Design review of the part built by this model. Coordinates are the model's own, in mm. A direction names the side the tool comes from. Give positions to 0.01 mm unless a question says otherwise; leave off trailing zeros. Order: outer loops, then holes, each group sorted by start corner. A loop starts at its lowest first (then second) coordinate and runs counter-clockwise, first axis right, second up. Notation, with made-up numbers: (83, 28) -> (121, 28) arc R17 ccw to (121, 49) -> close; hole circle Ø8 at (26, 17). An arc over 180 degrees is marked (long way). One line per item, written item: value. Start each with the question number.
1) Tool access review of faces 3 (the face through (-72.563, -93.809, 13.957)), 4 (the face through (-19.567, 101.123, 20.944)): name each direction out of +Z, -Z, +X, -X, +Y, -Y from which nothing blocks a thin tool from reaching the whole face with its end or side.
2) Consider section A-A (x = 0). State the section outline as (y, z) points, plus the area to 3 significant figures.
3) Consider section B-B (y = 55). State the section outline as (x, z) points.
4) Wall thickness on line 1 along Y through (x, z) = (0, 12.25); line 2 along X through (y, z) = (-3, 4); line 3 along Y through (x, z) = (-20, 10.5): over which ranges is each line inside the solid? List them lowest first. Write a range as from..to.
5) The part is to be moulded in two halves that separate along Y. For faces 1 (the face through (77, -57, 25)), 2 (the face through (-68.887, -95.472, 13.957)), say which applies: released by +Y, released by -Y, zero draft, split by the parting line, or undercut.
6) Consider section C-C (z = 20.5). State how many separate pieces and enclosed holes the cut face has, plus the area to 3 significant figures.
7) For pin 1 (1 mm diameter, centred on y = 51, z = 12.5, fed in from -X); pin 2 (1.5 mm diameter, centred on x = -91, z = 15.5, fed in from +Y); pin 3 (12 mm diameter, centred on y = -37, z = 8, fed in from -X); pin 4 (5 mm diameter, centred on x = -95.26, y = -55, fed in from -Z), all flat-tipped, find the tip position at first contact; note any pin that passes through.
from build123d import *

# Parameters (mm, degrees)
F2_START      = 2
F0_R          = 4.2
F0_R_2        = 95
F2_DEPTH      = 23
F4_DEPTH      = 35
F4_DEPTH_BACK = 10
F5_COUNT      = 6
F8_DEPTH      = 8
F8_DEPTH_BACK = 10
F9_COUNT      = 6
F12_D         = 5
F12_DEPTH     = 12
F12_START     = 2
F12_TIP       = 1.5021515476
F13_SIZE      = 0.6


with BuildPart() as f2:
    # F0 (on Top) → F2 (new body)
    with BuildSketch(Plane.XY.offset(F2_START)):
        Polygon((75, 129.9038105677), (-75, 129.9038105677), (-150, 0), (-75, -129.9038105677), (75, -129.9038105677), (150, 0), align=None)
        with Locations((-95.2627944163, -55)):
            Circle(F0_R, mode=Mode.SUBTRACT)
        with Locations((0, -110)):
            Circle(F0_R, mode=Mode.SUBTRACT)
        with Locations((95.2627944163, -55)):
            Circle(F0_R, mode=Mode.SUBTRACT)
        with Locations((-95.2627944163, 55)):
            Circle(F0_R, mode=Mode.SUBTRACT)
        Circle(F0_R_2, mode=Mode.SUBTRACT)
        with Locations((95.2627944163, 55)):
            Circle(F0_R, mode=Mode.SUBTRACT)
        with Locations((0, 110)):
            Circle(F0_R, mode=Mode.SUBTRACT)
    extrude(amount=F2_DEPTH)


with BuildPart() as f4:
    # F3 (on Top) → F4 (new body, two sides)
    with BuildSketch(Plane.XY) as f4_sk:
        with BuildLine():
            ThreePointArc((-34.5435296861, 77.6643068393), (-32.6327882373, 78.4863117484), (-30.7025049427, 79.2613158498))
            ThreePointArc((-30.7025049427, 79.2613158498), (-41.9019572207, 106.1559598637), (-65.2675230757, 123.5571075336))
            ThreePointArc((-65.2675230757, 123.5571075336), (-66.656996648, 123.5810891624), (-67.7266746593, 122.6939584625))
            ThreePointArc((-67.7266746593, 122.6939584625), (-67.8817545517, 121.0315856662), (-66.7217246277, 119.8308093913))
            ThreePointArc((-66.7217246277, 119.8308093913), (-44.7195832857, 103.2599332678), (-34.5435296861, 77.6643068393))
        make_face()
    extrude(amount=F4_DEPTH)
    extrude(f4_sk.sketch, amount=-F4_DEPTH_BACK)


with BuildPart() as f5_1:
    # F5: instance of F4
    add(f4.part.rotate(Axis((0, 0, -0.1854561269), (0, 0, 1)), 1 * 360 / F5_COUNT))


with BuildPart() as f5_2:
    # F5: instance of F4
    add(f4.part.rotate(Axis((0, 0, -0.1854561269), (0, 0, 1)), 2 * 360 / F5_COUNT))


with BuildPart() as f5_3:
    # F5: instance of F4
    add(f4.part.rotate(Axis((0, 0, -0.1854561269), (0, 0, 1)), 3 * 360 / F5_COUNT))


with BuildPart() as f5_4:
    # F5: instance of F4
    add(f4.part.rotate(Axis((0, 0, -0.1854561269), (0, 0, 1)), 4 * 360 / F5_COUNT))


with BuildPart() as f5_5:
    # F5: instance of F4
    add(f4.part.rotate(Axis((0, 0, -0.1854561269), (0, 0, 1)), 5 * 360 / F5_COUNT))


with BuildPart() as f2_1:
    add(f2.part)

    # F6: cut F4, F5_5, F5_4, F5_3, F5_2, F5_1
    add(f4.part, mode=Mode.SUBTRACT)
    add(f5_5.part, mode=Mode.SUBTRACT)
    add(f5_4.part, mode=Mode.SUBTRACT)
    add(f5_3.part, mode=Mode.SUBTRACT)
    add(f5_2.part, mode=Mode.SUBTRACT)
    add(f5_1.part, mode=Mode.SUBTRACT)

    # F9: F8 ×6 about axis
    f9_axis = Axis((0, 0, -0.1854561269), (0, 0, 1))


with BuildPart() as f8:
    # F7 (on face) → F8 (new body, two sides)
    with BuildSketch(Plane.XY.offset(25)) as f8_sk:
        with BuildLine():
            ThreePointArc((-14.9635818085, 97.9443271428), (-16.6533189284, 100.4972414515), (-19.6533265238, 101.1075998951))
            ThreePointArc((-19.6533265238, 101.1075998951), (-22.2062408325, 99.4178627752), (-22.8165992761, 96.4178551798))
            Line((-22.8165992761, 96.4178551798), (-20.6971664161, 85.5143183486))
            Line((-20.6971664161, 85.5143183486), (-16.7706576823, 86.2775543301))
            Line((-16.7706576823, 86.2775543301), (-12.8441489485, 87.0407903117))
            Line((-12.8441489485, 87.0407903117), (-14.9635818085, 97.9443271428))
        make_face()
    extrude(amount=-F8_DEPTH)
    extrude(f8_sk.sketch, amount=F8_DEPTH_BACK)


with BuildPart() as f2_2:
    add(f2_1.part)
    for i in range(1, F9_COUNT):
        add(f8.part.rotate(f9_axis, i * 360 / F9_COUNT), mode=Mode.SUBTRACT)

    # F9#seed: cut F8
    add(f8.part, mode=Mode.SUBTRACT)

    # F12
    # its depths count from where the whole tool has entered the part; down to there all is cleared
    with Locations(Plane(origin=(0, 0, 0), x_dir=(1, 0, 0), z_dir=(0, 0, -1)).offset(-F12_START)):
        with Locations((-85.2627944163, -72.3205080757), (20, -110), (105.2627944163, -37.6794919243), (85.2627944163, 72.3205080757), (-20, 110), (-105.2627944163, 37.6794919243)):
            Hole(F12_D / 2, depth=F12_DEPTH)
            with Locations((0, 0, -(F12_DEPTH + F12_TIP / 2))):  # 118° drill point
                Cone(0, F12_D / 2, F12_TIP, mode=Mode.SUBTRACT)

    # F13
    f13_edges = [f2_2.edges().sort_by_distance(p)[0] for p in [
        (48.019062, -107.161639, 2),
        (116.814232, -11.995092, 2),
        (68.79517, 95.166547, 2),
        (-48.019062, 107.161639, 2),
        (-116.814232, 11.995092, 2),
        (-68.79517, -95.166547, 2),
    ]]
    chamfer(f13_edges, length=F13_SIZE)


solid = f2_2.part
Checked values:
1. face 3: +Z, -Z
1. face 4: +Z
2. outline: (-129.9, 2) -> (-114.2, 2) -> (-114.2, 25) -> (-129.9, 25) -> close; (-105.8, 2) -> (-95, 2) -> (-95, 25) -> (-105.8, 25) -> close; (95, 2) -> (105.8, 2) -> (105.8, 25) -> (95, 25) -> close; (114.2, 2) -> (129.9, 2) -> (129.9, 25) -> (114.2, 25) -> close
2. area: 1,220 mm^2
3. outline: (-118.25, 2) -> (-99.46, 2) -> (-99.46, 25) -> (-118.25, 25) -> close; (-91.06, 2) -> (-77.46, 2) -> (-77.46, 25) -> (-91.06, 25) -> close; (77.46, 2) -> (91.06, 2) -> (91.06, 25) -> (77.46, 25) -> close; (99.46, 2) -> (118.25, 2) -> (118.25, 25) -> (99.46, 25) -> close
4. line 1: y = -129.9..-114.2, -105.8..-95, 95..105.8, 114.2..129.9
4. line 2: x = -148.27..-94.95, 94.95..136.02, 140.26..148.27
4. line 3: y = -129.9..-112.5, -107.5..-92.87, 92.87..129.9
5. face 1: zero draft
5. face 2: undercut
6. separate pieces: 1
6. enclosed holes: 7
6. area: 28,300 mm^2
7. pin 1: stops at x = -120.84
7. pin 2: stops at y = 103.49
7. pin 3: stops at x = -132.1
7. pin 4: passes through
